```python
from build123d import *

# Parameters (mm, degrees)
F1_DEPTH = 50
F2_R     = 12
F3_DEPTH = 5
F4_R     = 6.35
F5_DEPTH = 28
F6_W     = 36.939165
F6_H     = 22.77072
F7_DEPTH = 19
F8_R     = 1.35
F9_DEPTH = 31.001


with BuildPart() as f1:
    # F0 (on Top) → F1 (new body)
    with BuildSketch(Plane.XY):
        with BuildLine():
            Line((-38.126156, 8.452365), (-20, 0))
            Line((-20, 0), (20, 0))
            Line((20, 0), (38.126156, 8.452365))
            ThreePointArc((38.126156, 8.452365), (40.804064, 16.859756), (32.20674, 18.845061))
            ThreePointArc((32.20674, 18.845061), (0, 10.761955), (-32.20674, 18.845061))
            ThreePointArc((-32.20674, 18.845061), (-40.804064, 16.859756), (-38.126156, 8.452365))
        make_face()
    extrude(amount=F1_DEPTH)

    # F2 (on face) → F3 (join)
    with BuildSketch(Plane.XZ):
        with Locations((0, 25)):
            Circle(F2_R)
    extrude(amount=F3_DEPTH)

    # F4 (on face) → F5 (join)
    with BuildSketch(Plane.XZ.offset(5)):
        with Locations((0, 25)):
            Circle(F4_R)
    extrude(amount=F5_DEPTH)

    # F6 (on face) → F7 (cut)
    with BuildSketch(Plane.XY.offset(50)):
        with Locations((0.371061, -36.38536)):
            Rectangle(F6_W, F6_H)
    extrude(amount=-F7_DEPTH, mode=Mode.SUBTRACT)

    # F8 (on face) → F9 (cut, through all)
    with BuildSketch(Plane.XY.offset(31)):
        with Locations((0, -28)):
            Circle(F8_R)
    extrude(amount=-F9_DEPTH, mode=Mode.SUBTRACT)


solid = f1.part
```
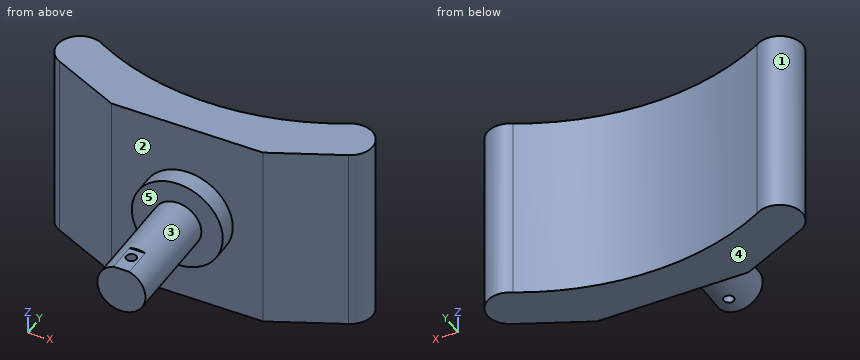
Geometry check sheet. Reference: the model listing, model coordinates, mm. Face numbers are marked on the shaded views. A direction names the side the tool comes from. Coordinates: 2 decimals unless noted, no trailing zeros. Order: outer loops, then holes, each group sorted by start corner. A loop starts at its lowest first (then second) coordinate and runs counter-clockwise, first axis right, second up. Notation, with made-up numbers: (63, -8) - (122, -8) arc R30 ccw to (122, 19) - close; hole circle Ø1 at (88, 83.5). An arc over 180 degrees is marked (long way). Answer as a JSON object with one key per item and string values. Group by question number.
Item 1: Sectioned sample at A-A, the plane z = 25. Record the cut outline in (x, y), and give its area (3 significant figures).
Item 2: Scan lines: probe 1 along Y at (x, z) = (0, 28); probe 2 along X at (y, z) = (-28, 27); probe 3 along Y at (x, z) = (33, 30). Record each from-to range of solid material in increasing order.
Item 3: Draft check along X on the marked faces 1, 2 and 3. Enter one of: +X half, -X half, draft (parallel to the pull), parting line (faces both ways), or undercut.
Item 4: Tool access check on the marked faces 4 and 5. Record the directions out of +Z, -Z, +X, -X, +Y, -Y that give a thin tool (end or side, any length) a straight path to the whole face; none if there is none.
Item 5: Sectioned sample at D-D, the plane z = 38.5. Record the cut outline in (x, y).
Item 6: Sectioned sample at B-B, the plane x = 0. Record the cut outline in (y, z), and give its area (3 significant figures).
Item 7: Sectioned sample at C-C, the plane y = -28. Record the cut outline in (x, z).
Item 8: Depth check by flat-ended pin: pin 1 Ø8 at (x, z) = (19.5, 19.5) entering from -Y; pin 2 Ø6 at (x, y) = (-18.5, -5.5) entering from -Z; pin 3 Ø10 at (y, z) = (5, 10.5) entering from +X; pin 4 Ø8 at (y, z) = (-8.5, 24.5) entering from +X. Enter the tip coordinate at first touch or a pass-through.
Resolved:
{
 "1": {"outline": "(-38.13, 8.45) - (-20, 0) - (-12, 0) - (-12, -5) - (-6.35, -5) - (-6.35, -33) - (6.35, -33) - (6.35, -5) - (12, -5) - (12, 0) - (20, 0) - (38.13, 8.45) arc R6 ccw (long way) to (32.21, 18.85) arc R68.2 cw to (-32.21, 18.85) arc R6 ccw (long way) to start; hole circle Ø2.7 at (0, -28)", "area": "1,470 mm^2"},
 "2": {"probe 1": "-33 to -29.35, -26.65 to 10.76", "probe 2": "-6.03 to -1.35, 1.35 to 6.03", "probe 3": "6.06 to 19.3"},
 "3": {"face 1": "undercut", "face 2": "draft", "face 3": "parting line"},
 "4": {"face 4": "-Z, +X, -X, +Y, -Y", "face 5": "-Y"},
 "5": {"outline": "(-38.13, 8.45) - (-20, 0) - (20, 0) - (38.13, 8.45) arc R6 ccw (long way) to (32.21, 18.85) arc R68.2 cw to (-32.21, 18.85) arc R6 ccw (long way) to start"},
 "6": {"outline": "(-33, 18.65) - (-29.35, 18.65) - (-29.35, 31) - (-33, 31) - close; (-26.65, 18.65) - (-5, 18.65) - (-5, 13) - (0, 13) - (0, 0) - (10.76, 0) - (10.76, 50) - (0, 50) - (0, 37) - (-5, 37) - (-5, 31.35) - (-25, 31.35) - (-25, 31) - (-26.65, 31) - close", "area": "978 mm^2"},
 "7": {"outline": "(-2.08, 31) arc R6.35 ccw to (-1.35, 18.8) - (-1.35, 31) - close; (1.35, 18.8) arc R6.35 ccw to (2.08, 31) - (1.35, 31) - close"},
 "8": {"pin 1": "y = 0", "pin 2": "through", "pin 3": "x = 40.16", "pin 4": "x = 12"}
}
